Here's how the part is built. I have some questions about the finished solid (model axes, mm). A direction names the side the tool comes from. Coordinates: 2 decimals unless noted, no trailing zeros. Write each loop counter-clockwise with the first axis right and the second up, starting at its lowest first coordinate (ties: lowest second). Pieces come first, ordered by that corner, then holes. Notation, with made-up numbers: (59, 16.25) -> (73, 16.25) arc R31 cw to (73, 42.25) -> close; hole circle Ø11 at (12, 81). An arc over 180 degrees is marked (long way). Use a Markdown table: item, result. Add a question column.
Item 1: Imagine slicing it at B-B, the plane y = 45.5. Write out the boundary of the cut face in (x, z), and give its area (3 significant figures).
Item 2: On a 3-axis mill with a long thin cutter (end or side, diameter ignored), from which of +Z, -Z, +X, -X, +Y, -Y can I reach the whole of each face in a straight line? I mean faces 5 (the cylindrical face through (8.75, 43.36, 0.17)), 6 (the flat face through (8.4, 45.892, 0)). Say none if no direction works.
Item 3: Imagine slicing it at D-D, the plane y = 37. Write out the boundary of the cut face in (x, z), and give its area (3 significant figures).
Item 4: If I drill on line 1 along X through (y, z) = (40, 0); line 2 along Y through (x, z) = (7.25, -5.75); line 3 along Z through (x, y) = (6, 41.5), over which ranges is the centre line in solid material (lowest first)? Write a range as from..to.
Item 5: If we mould it in two halves opening along X, with no side actions, what happens to faces 1 (the flat face through (-7, 35.892, -4.3)), 2 (the cylindrical face through (-8.75, 43.36, -0.17)), 3 (the cylindrical face through (-3.06, 40.82, 7.39)), 4 (the cylindrical face through (-5.78, 38.36, -7.54))? For each: pulls with the +X half, pulls with the -X half, needs draft (parallel to the pull), parting line crosses it, or undercut.
Item 6: Will these pins go through, and if not, where does the flat tip stop? pin 1 Ø6 at (x, y) = (3.5, 37.5) entering from +Z; pin 2 Ø0.8 at (y, z) = (43.5, 8) entering from +X; pin 3 Ø3 at (y, z) = (44.5, 4.5) entering from -X.
Item 7: Imagine slicing it at C-C, the plane z = 0. Write out the boundary of the cut face in (x, y).
Item 8: Imagine slicing it at A-A, the plane x = 0. Write out the boundary of the cut face in (y, z), and give its area (3 significant figures).
```python
from build123d import *

# Parameters (mm, degrees)
SKETCH1_R               = 95
SKETCH1_R_2             = 80
BOSS_EXTRUDE1_DEPTH     = 50
SKETCH2_R               = 87.5
SKETCH2_R_2             = 80
BOSS_EXTRUDE2_DEPTH     = 50
CUT_EXTRUDE1_DEPTH      = 168.481342244
CUT_EXTRUDE1_DEPTH_BACK = 168.481342244
SCALE1_SCALE            = 0.1


with BuildPart() as part:
    # Sketch1 → Boss-Extrude1 (new body)
    with BuildSketch(Plane(origin=(0, 0, 0), x_dir=(1, 0, 0), z_dir=(0, 1, 0))):
        with Locations(Location((0, 0, 0), (0, 0, 270))):
            Circle(SKETCH1_R)
        with Locations(Location((0, 0, 0), (0, 0, 270))):
            Circle(SKETCH1_R_2, mode=Mode.SUBTRACT)
    extrude(amount=BOSS_EXTRUDE1_DEPTH)

    # Sketch2 → Boss-Extrude2 (add)
    with BuildSketch(Plane(origin=(0, 50, 0), x_dir=(1, 0, 0), z_dir=(0, 1, 0))):
        with Locations(Location((0, 0, 0), (0, 0, 270))):
            Circle(SKETCH2_R)
        with Locations(Location((0, 0, 0), (0, 0, 270))):
            Circle(SKETCH2_R_2, mode=Mode.SUBTRACT)
    extrude(amount=BOSS_EXTRUDE2_DEPTH)

    # Sketch4 → Cut-Extrude1 (cut, two sides: drawn at the far end of the back side and taken through both)
    with BuildSketch(Plane.XY.offset(-CUT_EXTRUDE1_DEPTH_BACK)):
        Polygon((0, 100), (-15, 100), (-15, 50), (15, 50), (15, 100), align=None)
    extrude(amount=CUT_EXTRUDE1_DEPTH + CUT_EXTRUDE1_DEPTH_BACK, mode=Mode.SUBTRACT)


with BuildPart() as part_1:
    # Scale1: scaled about (0, 39.880423453, 0)
    add(part.part.scale(SCALE1_SCALE).moved(Location((0, 35.892381108, 0))))


solid = part_1.part
```
Ans:
| question | item | result |
|---|---|---|
| 1 | outline | (-1.5, -8.62) -> (-1.5, -7.86) arc R8 cw to (-1.5, 7.86) -> (-1.5, 8.62) arc R8.75 ccw to start; (1.5, -8.62) arc R8.75 ccw to (1.5, 8.62) -> (1.5, 7.86) arc R8 cw to (1.5, -7.86) -> close |
| 1 | area | 34.9 mm^2 |
| 2 | face 5 | +X, +Y |
| 2 | face 6 | +Z, -Z, +X, -X, +Y |
| 3 | outline | circle Ø19 at (0, 0); hole circle Ø16 at (0, 0) |
| 3 | area | 82.5 mm^2 |
| 4 | line 1 | x = -9.5..-8, 8..9.5 |
| 4 | line 2 | y = 35.89..40.89 |
| 4 | line 3 | z = -6.37..-5.29, 5.29..6.37 |
| 5 | face 1 | needs draft |
| 5 | face 2 | pulls with the -X half |
| 5 | face 3 | undercut |
| 5 | face 4 | parting line crosses it |
| 6 | pin 1 | stops at z = 9.49 |
| 6 | pin 2 | stops at x = 4.34 |
| 6 | pin 3 | stops at x = -8.22 |
| 7 | outline | (-9.5, 35.89) -> (-8, 35.89) -> (-8, 45.89) -> (-8.75, 45.89) -> (-8.75, 40.89) -> (-9.5, 40.89) -> close; (8, 35.89) -> (9.5, 35.89) -> (9.5, 40.89) -> (8.75, 40.89) -> (8.75, 45.89) -> (8, 45.89) -> close |
| 8 | outline | (35.89, -9.5) -> (40.89, -9.5) -> (40.89, -8) -> (35.89, -8) -> close; (35.89, 8) -> (40.89, 8) -> (40.89, 9.5) -> (35.89, 9.5) -> close |
| 8 | area | 15.0 mm^2 |
